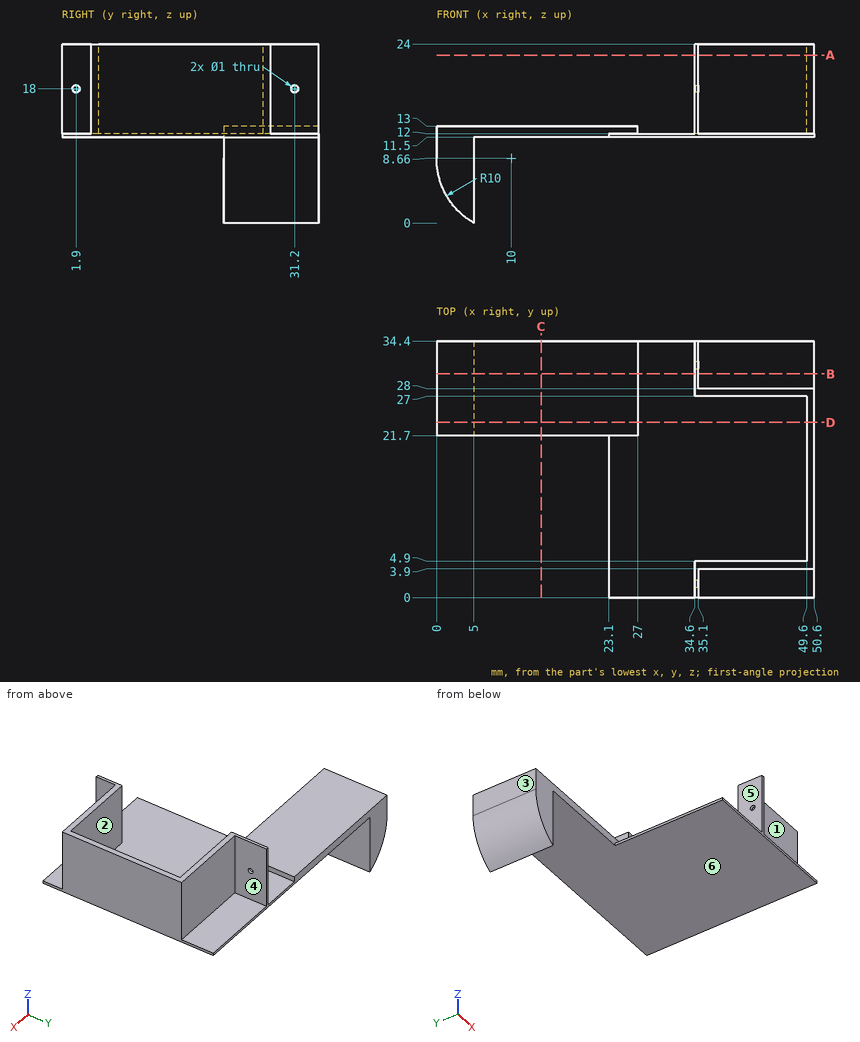
Verification items for this drawing (mm, ordinates from the low corner). A direction names the side the tool comes from. Coordinates: 2 decimals unless noted, no trailing zeros. Loops run counter-clockwise (first coordinate to the right, second up) from the corner with the lowest first, then second, coordinate; pieces in that order, holes last. Notation, with made-up numbers: (-39.5, 87) -> (-32.5, 87) arc R20 cw to (-32.5, 98) -> close; hole circle Ø5 at (4, 71.5). An arc over 180 degrees is marked (long way). Answer in a Markdown table with one row per item. Add a question column.
1. Section check D-D, the plane y = 23.5. Enter the section's corners in (x, z), then the cut area to 3 significant figures.
2. Section check B-B, the plane y = 30. Enter the section's corners in (x, z).
3. Section check A-A, the plane z = 22.5. Enter the section's corners in (x, y).
4. Access from +Z, -Z, +X, -X, +Y, -Y to the whole of each face (thin tool, end or side, straight path). Record for the marked faces 4, 5 and 6.
5. Depth check by flat-ended pin: P1, Ø1.9, axis at x = 43, y = 32, coming from the +Z side; P2, Ø2, axis at y = 12, z = 14.5, coming from the -X side; P3, Ø1, axis at y = 31, z = 7.5, coming from the +X side. Enter the tip coordinate at first touch or a pass-through.
6. Material ranges on probe 1 along Y at (x, z) = (34.95, 18); probe 2 along Y at (x, z) = (41, 22); probe 3 along Z at (x, y) = (34.9, 1.9), recorded low to high. Write a range as [from, to].
7. Draft check along Y on the marked faces 1, 2 and 3. Enter one of: +Y half, -Y half, draft (parallel to the pull), parting line (faces both ways), or undercut.
8. Section check C-C, the plane x = 14. Enter the section's corners in (y, z).
Derived:
| question | item | result |
|---|---|---|
| 1 | outline | (0, 8.66) arc R10 ccw to (5, 0) -> (5, 11.5) -> (50.6, 11.5) -> (50.6, 24) -> (49.6, 24) -> (49.6, 12) -> (27, 12) -> (27, 13) -> (0, 13) -> close |
| 1 | area | 109 mm² |
| 2 | outline | (0, 8.66) arc R10 ccw to (5, 0) -> (5, 11.5) -> (50.6, 11.5) -> (50.6, 12) -> (35.1, 12) -> (35.1, 24) -> (34.6, 24) -> (34.6, 12) -> (27, 12) -> (27, 13) -> (0, 13) -> close |
| 3 | outline | (34.6, 0) -> (35.1, 0) -> (35.1, 3.9) -> (50.6, 3.9) -> (50.6, 28) -> (35.1, 28) -> (35.1, 34.4) -> (34.6, 34.4) -> (34.6, 27) -> (49.6, 27) -> (49.6, 4.9) -> (34.6, 4.9) -> close |
| 4 | face 4 | +Z, +X, +Y |
| 4 | face 5 | +Z, -X, +Y, -Y |
| 4 | face 6 | -Z, +X, +Y, -Y |
| 5 | P1 | stops at z = 12 |
| 5 | P2 | stops at x = 49.6 |
| 5 | P3 | stops at x = 5 |
| 6 | probe 1 | y = [0, 1.4], [2.4, 4.9], [27, 30.7], [31.7, 34.4] |
| 6 | probe 2 | y = [3.9, 4.9], [27, 28] |
| 6 | probe 3 | z = [11.5, 17.5], [18.5, 24] |
| 7 | face 1 | -Y half |
| 7 | face 2 | undercut |
| 7 | face 3 | draft |
| 8 | outline | (21.7, 11.5) -> (34.4, 11.5) -> (34.4, 13) -> (21.7, 13) -> close |
